Autodesk Inventor part; units mm, degrees
ref_plane "YZ Plane" through (0, 0, 0) normal (1, 0, 0) x (0, 1, 0)
ref_plane "XZ Plane" through (0, 0, 0) normal (0, 1, 0) x (-1, 0, 0)
ref_plane "XY Plane" through (0, 0, 0) normal (0, 0, 1) x (1, 0, 0)
sketch "スケッチ1" plane through (0, 0, 0) normal (0, 0, 1) x (1, 0, 0)
  circle A0 centre (0, 0) radius 5.025
  circle A1 centre (0, 0) radius 10
  line L0 (0, 0) -> (14.1421, -14.1421)
  line L1 (0, 0) -> (20, 0) construction
  line L2 (0, 0) -> (14.1421, -14.1421) construction
  line L3 (-7.0711, -7.0711) -> (7.0711, -21.2132)
  line L4 (21.2132, -7.0711) -> (7.0711, 7.0711)
  arc A2 (7.0711, 7.0711) -> (-7.0711, -7.0711) centre (0, 0) ccw
  arc A3 (7.0711, -21.2132) -> (21.2132, -7.0711) centre (14.1421, -14.1421) ccw
  circle A4 centre (14.1421, -14.1421) radius 4.025
  circle A5 centre (14.1421, -14.1421) radius 13
  circle A6 centre (14.1421, -14.1421) radius 14
  line L5 (4.2426, -24.0416) -> (21.0227, -40.8217)
  line L6 (21.0227, -40.8217) -> (47.0109, -27.2119)
  line L7 (47.0109, -27.2119) -> (24.0416, -4.2426)
  arc A7 (12.0122, -27.9792) -> (10.7234, -30.5224) centre (11.784, -29.4617) ccw
  line L8 (-8.3867, -5.4464) -> (8.8712, -32.0212)
  arc A8 (10.5855, -29.4018) -> (10.585, -29.4134) centre (11.784, -29.4617) ccw
  line L9 (4.2426, -24.0416) -> (21.0227, -40.8217)
  line L10 (21.0227, -40.8217) -> (47.0109, -27.2119)
  line L11 (47.0109, -27.2119) -> (24.0416, -4.2426)
  arc A9 (8.8712, -32.0212) -> (10.7228, -30.5218) centre (9.8758, -31.3688) ccw
  arc A10 (11.5527, -27.9797) -> (10.7228, -30.5218) centre (11.784, -29.4617) ccw
  arc A11 (11.5527, -27.9797) -> (23.9469, -16.1083) centre (9.2397, -13.1591) ccw
  arc A12 (-9.9898, 0.4505) -> (9.3407, -32.4405) centre (24.9746, -1.1263) ccw
  arc A13 (21.2132, -7.0711) -> (7.0711, -21.2132) centre (14.1421, -14.1421) ccw
  arc A14 (7.4956, -0.2576) -> (12.25, -4.3228) centre (11.4932, -0.395) ccw
  circle A15 centre (0, 0) radius 7.5
  line L12 (5.3033, 5.3033) -> (0.6262, 9.9804)
  arc A16 (-3.1585, -21.9475) -> (11.5527, -27.9797) centre (9.1773, -12.8178) ccw
  point P0 (7.0711, -7.0711)
  point P1 (7.0711, 7.0711)
  point P2 (10.4941, -23.453)
  point P3 (-8.3867, -5.4464)
  point P4 (9.5568, -27.6782)
  point P5 (9.5574, -27.6666)
  point P6 (-9.9898, 0.4505)
  point P7 (10.7234, -30.5224)
  point P8 (11.5527, -27.9797)
  point P9 (9.2796, -3.7267)
  point P10 (0.6262, 9.9804)
  dimension "d0" = 10.05
  dimension "d1" = 20
  dimension "d2" = 20
  dimension "d3" = 45
  dimension "d6" = 8.05
  dimension "d7" = 26
  dimension "d8" = 1
  dimension "d9" = 1.5
  dimension "d14" = 0
  dimension "d15" = 0
  dimension "d17" = 15
  dimension "d18" = 168
  dimension "d19" = 35
  dimension "d20" = 4
  dimension "d21" = 15
extrude "押し出し1" add sketch "スケッチ1" along normal blind 3 contours A6 A15 | A6 A15 A5 L0 | L0 A5 A15 A6 | A5 A15 L0 | L0 A15 A5 | A15 A14 A6 | A6 A14 A5 A15 | A15 A5 A1 A6 | A6 A1 L12 A15 | A15 A5 A14 A1 L0 | L0 A1 A5 A15 | A6 L3 A1 | A1 A5 L3 A6 | A13 L3 A5 A1 | A1 A14 A13 | A13 A3 | L3 A6 L5 A16 L8 A1 | L3 A5 A11 A6 | A3 A11 A5 L3 | L8 A16 A12 A1 | A6 A11 A16 L5
properties part number "従動節"
Work out the finished part from the listing and answer in its coordinate system (mm). Coordinates: 2 decimals unless noted, no trailing zeros. Order: outer loops, then holes, each group sorted by start corner. A loop starts at its lowest first (then second) coordinate and runs counter-clockwise, first axis right, second up. Notation, with made-up numbers: (23.5, 35) - (40.5, 35) arc R20 ccw to (40.5, 49) - close; hole circle Ø7 at (18, 56.25). An arc over 180 degrees is marked (long way). Answer as a JSON object with one key per item and string values.
1. The mould has two halves that part along X. Classify faces 1 (the face through (-8.454, -11.497, 1.479)), 2 (the face through (8.932, -3.468, 1.479)), 3 (the face through (7, -13, 3)), 4 (the face through (19.71, -23.9, 1.48)): +X half, -X half, draft (parallel to the pull), parting line (faces both ways), or undercut.
Output values:
{"face 1": "-X half", "face 2": "undercut", "face 3": "draft", "face 4": "+X half"}
2. Find section C-C on y = -19. Determine the outline of the cut face in (x, z), plus the area to 3 significant figures.
Output values:
{"outline": "(-5.12, 0) - (23.06, 0) - (23.06, 3) - (-5.12, 3) - close", "area": "84.5 mm²"}
3. Find section D-D on x = 22. Determine the outline of the cut face in (y, z).
Output values:
{"outline": "(-21.04, 0) - (-7.96, 0) - (-7.96, 3) - (-21.04, 3) - close"}
4. Each of these flat-tipped pins is pushed along its axis until it touches: P1, Ø9.5, axis at x = 14.14, y = -14.14, coming from the -Z side; P2, Ø3, axis at x = 12.5, y = -16, coming from the +Z side. Where does it stop, or does it pass through?
Output values:
{"P1": "stops at z = 0", "P2": "passes through"}
5. Consider line 1 (X direction, y = 4, z = 2.65); line 2 (Y direction, x = -2, z = 0.4); line 3 (Y direction, x = 13, z = 2.8). Determine where each line is inside the solid, lowest interval first.
Output values:
{"line 1": "x = -9.17 to -3.04, 3.04 to 6.34", "line 2": "y = -23.33 to -4.61, 4.61 to 9.8", "line 3": "y = -27.68 to -18, -10.28 to -4.21"}
6. Find section B-B on z = 1.7. Count the separate pieces of the cut face and the enclosed holes in it, plus the area to 3 significant figures.
Output values:
{"separate pieces": "1", "enclosed holes": "2", "area": "714 mm²"}
7. Find section A-A on x = -1.5. Determine the outline of the cut face in (y, z), plus the area to 3 significant figures.
Output values:
{"outline": "(-23.84, 0) - (-4.8, 0) - (-4.8, 3) - (-23.84, 3) - close; (4.8, 0) - (9.89, 0) - (9.89, 3) - (4.8, 3) - close", "area": "72.4 mm²"}
